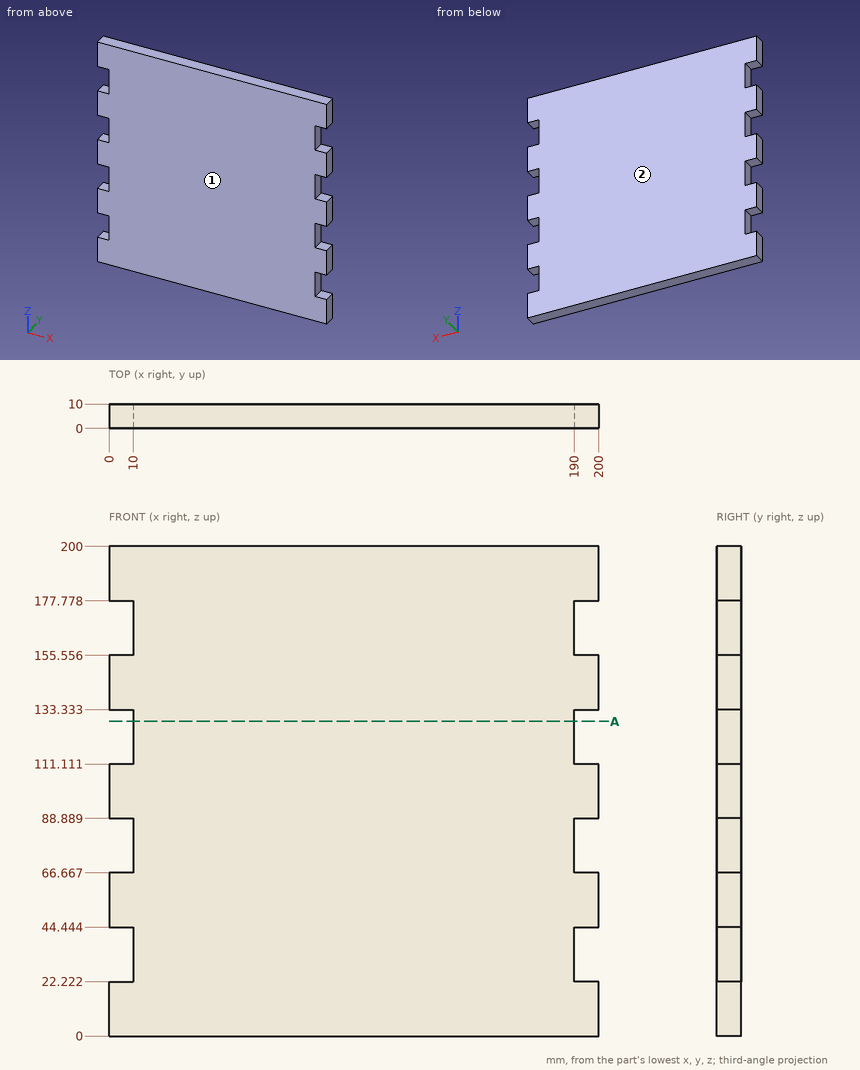
The drawing under review shows one solid part. Ordinate dimensions are in mm from its lowest x, y, z. Give positions to 0.01 mm unless a question says otherwise; leave off trailing zeros. Loops run counter-clockwise (first coordinate to the right, second up) from the corner with the lowest first, then second, coordinate; pieces in that order, holes last. Notation, with made-up numbers: M 44,35.25 L 90,35.25 A10 ccw 90,43.25 Z; hole C -30,75.25 d11. An arc over 180 degrees is marked long. Return JSON: item names as keys, results as strings. Group by question number.
Item 1: For probe 1 along X at (y, z) = (1.5, 165.5), list the stretches that pass through material, from the lowest coordinate up.
Item 2: We need section A-A (z = 128.5). Give the boundary of the cut face in (x, y), and give its area (3 significant figures).
Item 3: Mouldability with a two-part tool opening along Y and no side actions: class the marked faces 1 and 2 as released by +Y, released by -Y, zero draft, split by the parting line, or undercut.
Item 4: Insertion check: pin 1 Ø3 at (y, z) = (5, 26) entering from -X. The pin has a flat end and moves straight along its axis. Give the tip position at first contact, or say it passes through.
Output:
{
 "1": {"probe 1": "x = 10 to 190"},
 "2": {"outline": "M 10,0 L 190,0 L 190,10 L 10,10 Z", "area": "1,800 mm^2"},
 "3": {"face 1": "released by -Y", "face 2": "released by +Y"},
 "4": {"pin 1": "stops at x = 10"}
}
